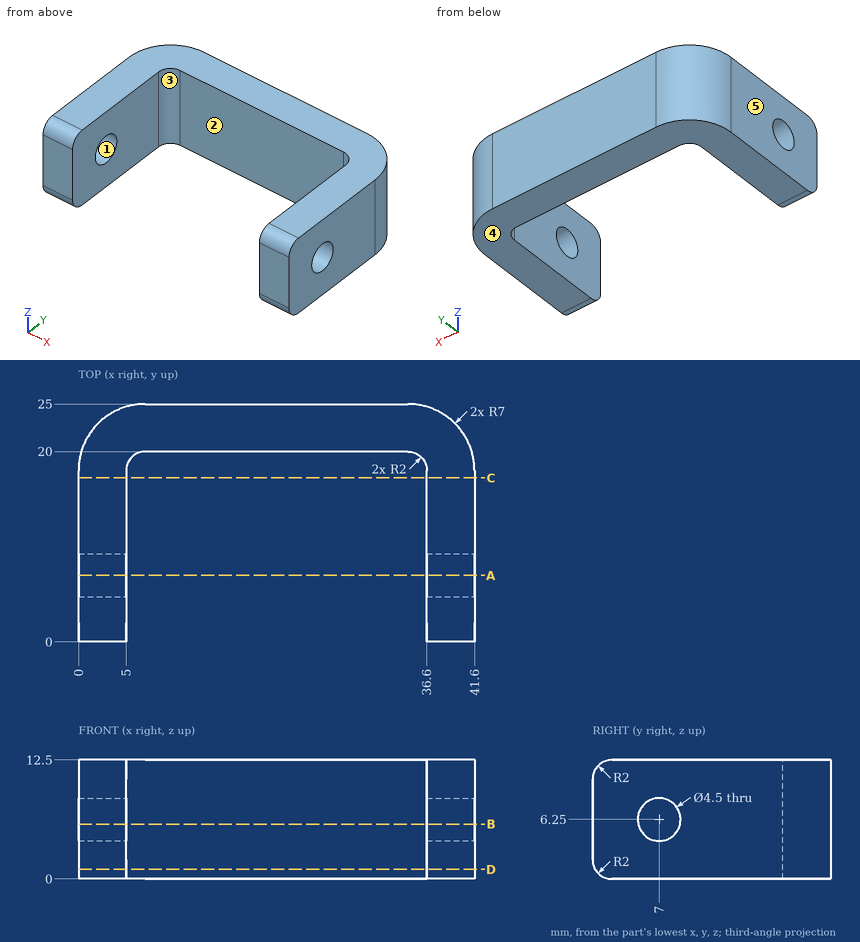
Design review of the part shown in the three views and the two pictorial views. Dimensions are in mm from the part's minimum x, y and z. A direction names the side the tool comes from. Give positions to 0.01 mm unless a question says otherwise; leave off trailing zeros. Loops run counter-clockwise (first coordinate to the right, second up) from the corner with the lowest first, then second, coordinate; pieces in that order, holes last. Notation, with made-up numbers: (37.5, 39) - (42.5, 39) arc R25 ccw to (42.5, 54) - close; hole circle Ø10 at (17, -8). An arc over 180 degrees is marked (long way). Answer as a JSON object with one key per item and string values.
Q1. Add section A-A on y = 7. State the section outline as (x, z) points, plus the area to 3 significant figures.
Worked out:
{"outline": "(0, 0) - (5, 0) - (5, 4) - (0, 4) - close; (0, 8.5) - (5, 8.5) - (5, 12.5) - (0, 12.5) - close; (36.6, 0) - (41.6, 0) - (41.6, 4) - (36.6, 4) - close; (36.6, 8.5) - (41.6, 8.5) - (41.6, 12.5) - (36.6, 12.5) - close", "area": "80.0 mm^2"}
Q2. Mouldability with a two-part tool opening along X and no side actions: class the marked faces 3, 4 and 5 as +X half, -X half, draft (parallel to the pull), parting line (faces both ways), or undercut.
Worked out:
{"face 3": "undercut", "face 4": "draft", "face 5": "-X half"}
Q3. For the marked faces 1 and 2, list the 3-axis set-ups (+Z, -Z, +X, -X, +Y, -Y) from which the entire face can be reached by the end or side of a thin tool; tool diameter is ignored.
Worked out:
{"face 1": "+X, -X", "face 2": "+Z, -Z, -Y"}
Q4. To check wall thickness, follow line 1 along X through (y, z) = (4.5, 9.25); line 2 along Y through (x, z) = (37.7, 6.25); line 3 along Y through (x, z) = (2.7, 6.25). State the ranges of each line that lie inside material, in increasing order.
Worked out:
{"line 1": "x = 0 to 5, 36.6 to 41.6", "line 2": "y = 0 to 4.75, 9.25 to 24.28", "line 3": "y = 0 to 4.75, 9.25 to 23.52"}
Q5. Add section C-C on y = 17.25. State the section outline as (x, z) points, plus the area to 3 significant figures.
Worked out:
{"outline": "(0, 0) - (5, 0) - (5, 12.5) - (0, 12.5) - close; (36.6, 0) - (41.6, 0) - (41.6, 12.5) - (36.6, 12.5) - close", "area": "125 mm^2"}
Q6. Insertion check: pin 1 (4 mm diameter, centred on x = 23.5, z = 9, fed in from -Y); pin 2 (2.5 mm diameter, centred on y = 7, z = 6.25, fed in from +X); pin 3 (1 mm diameter, centred on y = 22, z = 6, fed in from +X). Each pin has a flat end and moves straight along its axis. Give the tip position at first contact, or say it passes through.
Worked out:
{"pin 1": "stops at y = 20", "pin 2": "passes through", "pin 3": "stops at x = 40.66"}
Q7. Add section B-B on z = 5.75. State the section outline as (x, y) points.
Worked out:
{"outline": "(0, 0) - (5, 0) - (5, 4.81) - (0, 4.81) - close; (0, 9.19) - (5, 9.19) - (5, 18) arc R2 cw to (7, 20) - (34.6, 20) arc R2 cw to (36.6, 18) - (36.6, 9.19) - (41.6, 9.19) - (41.6, 18) arc R7 ccw to (34.6, 25) - (7, 25) arc R7 ccw to (0, 18) - close; (36.6, 0) - (41.6, 0) - (41.6, 4.81) - (36.6, 4.81) - close"}
Q8. Add section D-D on z = 1. State the section outline as (x, y) points.
Worked out:
{"outline": "(0, 0.27) - (5, 0.27) - (5, 18) arc R2 cw to (7, 20) - (34.6, 20) arc R2 cw to (36.6, 18) - (36.6, 0.27) - (41.6, 0.27) - (41.6, 18) arc R7 ccw to (34.6, 25) - (7, 25) arc R7 ccw to (0, 18) - close"}
